Part model, mm, in its own coordinate system. Round coordinates to 2 decimals unless told otherwise and drop trailing zeros. Loops run counter-clockwise (first coordinate to the right, second up) from the corner with the lowest first, then second, coordinate; pieces in that order, holes last.
Autodesk Inventor part; units mm, degrees
ref_plane "YZ Plane" through (0, 0, 0) normal (1, 0, 0) x (0, 1, 0)
ref_plane "XZ Plane" through (0, 0, 0) normal (0, 1, 0) x (-1, 0, 0)
ref_plane "XY Plane" through (0, 0, 0) normal (0, 0, 1) x (1, 0, 0)
sketch "Sketch1" plane through (0, 0, 0) normal (0, 0, 1) x (1, 0, 0)
  line L0 (0, 0) -> (63.5, 0)
  line L1 (63.5, 0) -> (63.5, -25.4)
  line L2 (63.5, -25.4) -> (0, -25.4)
  line L3 (0, -25.4) -> (0, 0)
  dimension "d0" = 63.5
  dimension "d1" = 25.4
extrude "Extrusion1" add sketch "Sketch1" along normal blind 76.2
sketch "Sketch2" plane through (0, 0, 0) normal (0, 1, 0) x (1, 0, 0)
  circle A0 centre (13.1221, -13.5403) radius 1.6574
  circle A1 centre (13.1221, -13.5403) radius 3.1433
  circle A2 centre (13.1221, -13.5403) radius 2.794
  point P0 (0, 0)
  point P1 (22.0121, -13.5403)
  point P2 (35.874, -13.5403)
  point P3 (13.1221, -22.4303)
  point P4 (22.0121, -22.4303)
  point P5 (13.1221, -22.4303)
  dimension "d4" = 3.3147
  dimension "d5" = 6.2865
  dimension "d6" = 5.588
  dimension "d22" = 8.89
  dimension "d23" = 8.89
  dimension "d24" = 8.89
extrude "Extrusion2" cut sketch "Sketch2" against normal blind 19.812 contours A0
extrude "Extrusion3" cut sketch "Sketch2" against normal blind 9.398 contours A2
extrude "Extrusion4" cut sketch "Sketch2" against normal blind 4.1148 contours A1
fillet "Fillet1" [suppressed]
loft "Loft1" [suppressed]
properties part number "Thermocyler_Block_Test"
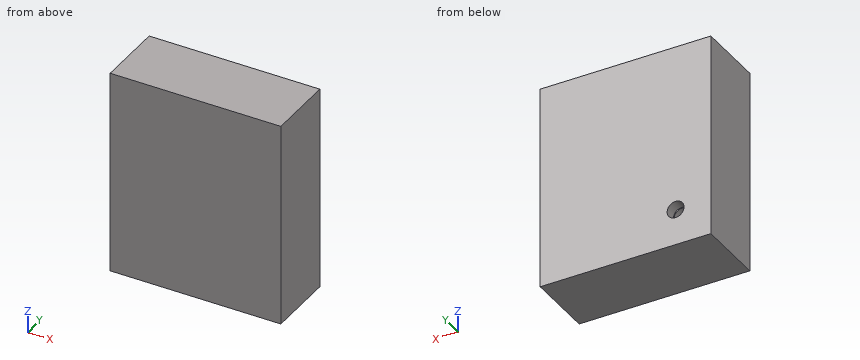
1) Slice it at A-A, the plane x = 13. Give the cut face in (y, z), then the cut area to 3 significant figures.
Values:
outline: (-25.4, 0) - (0, 0) - (0, 10.4) - (-4.11, 10.4) - (-4.11, 10.75) - (-9.4, 10.75) - (-9.4, 11.89) - (-19.81, 11.89) - (-19.81, 15.19) - (-9.4, 15.19) - (-9.4, 16.33) - (-4.11, 16.33) - (-4.11, 16.68) - (0, 16.68) - (0, 76.2) - (-25.4, 76.2) - close
area: 1,850 mm2
2) Wall check: line 1 along X through (y, z) = (-14.5, 15); line 2 along X through (y, z) = (-8.75, 11); line 3 along Z through (x, y) = (12, -8.25). Give the ranges that are in metal, low to high.
Values:
line 1: x = 0 to 12.34, 13.91 to 63.5
line 2: x = 0 to 11.96, 14.29 to 63.5
line 3: z = 0 to 10.98, 16.1 to 76.2
3) Drop flat-ended pins along their axis: pin 1 Ø5 at (x, z) = (13.12, 13.54) entering from +Y; pin 2 Ø2.5 at (x, z) = (13, 13.5) entering from +Y; pin 3 Ø5 at (x, z) = (13, 14) entering from +Y. Give the stop position or say it passes through.
Values:
pin 1: stops at y = -9.4
pin 2: stops at y = -19.81
pin 3: stops at y = -4.11
